```python
from build123d import *

# Parameters (mm, degrees)
SKETCH_R     = 7.5
PAD_DEPTH    = 5
SKETCH001_R  = 5.1
POCKET_DEPTH = 4
CHAMFER_SIZE = 1


with BuildPart() as part:
    # Sketch → Pad (new body)
    with BuildSketch(Plane.XY):
        Circle(SKETCH_R)
    extrude(amount=-PAD_DEPTH)

    # Sketch001 → Pocket (cut)
    with BuildSketch(Plane.XY):
        Circle(SKETCH001_R)
    extrude(amount=-POCKET_DEPTH, mode=Mode.SUBTRACT)

    # Chamfer
    chamfer_edges = [part.edges().sort_by_distance(p)[0] for p in [
        (-5.1, 0, 0),
    ]]
    chamfer(chamfer_edges, length=CHAMFER_SIZE)


solid = part.part
```
Input: part model. Units: mm. Frame: model coordinates. A direction names the side the tool comes from. Give positions to 0.01 mm unless a question says otherwise; leave off trailing zeros. Order: outer loops, then holes, each group sorted by start corner. A loop starts at its lowest first (then second) coordinate and runs counter-clockwise, first axis right, second up. Notation, with made-up numbers: M 82,-24.75 L 133,-24.75 A16 ccw 133,4.25 Z; hole C 51,-23 d4. An arc over 180 degrees is marked long. Return JSON: item names as keys, results as strings.
Item 1: Cut plane C-C (z = -3.75). Return loops of the section in (x, y).
Solutions:
{"outline": "C 0,0 d15; hole C 0,0 d10.2"}
Item 2: Access query for faces 1 (the flat face through (0, 0, -4)), 2 (the flat face through (0, 0, -5)). Directions: +Z, -Z, +X, -X, +Y, -Y. A direction counts if a zero-diameter tool reaches every point of the face in a straight line with its end or side. Return the directions, or none.
Solutions:
{"face 1": "+Z", "face 2": "-Z, +X, -X, +Y, -Y"}
Item 3: Ray query, probe 1 along Y at (x, z) = (0, -2.75); probe 2 along Z at (x, y) = (4.5, -1.75); probe 3 along Y at (x, z) = (-1.5, -3.15). Return the intervals inside material, ascending.
Solutions:
{"probe 1": "-7.5 to -5.1, 5.1 to 7.5", "probe 2": "-5 to -4", "probe 3": "-7.35 to -4.87, 4.87 to 7.35"}
Item 4: Cut plane A-A (x = 0). Return loops of the section in (y, z), then the cut area to 3 significant figures.
Solutions:
{"outline": "M -7.5,-5 L 7.5,-5 L 7.5,0 L 6.1,0 L 5.1,-1 L 5.1,-4 L -5.1,-4 L -5.1,-1 L -6.1,0 L -7.5,0 Z", "area": "33.2 mm^2"}
Item 5: Pull-direction query (X, two-part tool) for faces 3 (the cylindrical face through (-7.493, 0.33, -2.465)), 4 (the flat face through (2, -6, 0)), 5 (the cylindrical face through (2.4, -4.5, -2.5)); classes: +X half, -X half, draft (parallel to the pull), parting line (faces both ways), or undercut.
Solutions:
{"face 3": "parting line", "face 4": "draft", "face 5": "undercut"}
Item 6: First-contact query: P1, Ø3, axis at x = 2, z = -1, coming from the -Y side; P2, Ø3, axis at y = -1.5, z = -4, coming from the -X side; P3, Ø1.5, axis at x = 3, z = -4, coming from the +Y side; P4, Ø6, axis at x = -1, y = 2.5, coming from the +Z side. Flat tips, straight axial feed; report the tip coordinate or a pass-through.
Solutions:
{"P1": "y = -7.48", "P2": "x = -7.5", "P3": "y = 7.15", "P4": "z = -0.41"}
